Read the model definition and answer for the solid it produces. Units are mm, in the model's axes. Give positions to 0.01 mm unless a question says otherwise; leave off trailing zeros. Loops run counter-clockwise (first coordinate to the right, second up) from the corner with the lowest first, then second, coordinate; pieces in that order, holes last. Notation, with made-up numbers: (82.5, 41.5) - (108.5, 41.5) arc R15 ccw to (108.5, 67.5) - close; hole circle Ø3 at (16.5, 10). An arc over 180 degrees is marked (long way). Put each result on its own line as item: value. Start each with the question number.
1. A cutting plane is placed at C-C, the plane z = 51. Determine the outline of the cut face in (x, y).
2. Consider L1, parallel to Y at x = 0, z = 20; L2, parallel to Y at x = -8, z = 52; L3, parallel to X at y = -11, z = 26. Determine where each line is inside the solid, lowest interval first. Write a range as from..to.
3. Given pin 1 Ø5 at (y, z) = (-16.5, 18) entering from -X; pin 2 Ø10 at (y, z) = (15.5, 41) entering from +X; pin 3 Ø10 at (y, z) = (16, 10.5) entering from -X; pin 4 Ø4 at (x, y) = (16, -17.5) entering from +Z, each flat-ended and moving along its own axis, determine where each tip first touches the part or whether it passes through.
4. For a pull along X with two mould halves and no side action, classify faces 1 (the cylindrical face through (-4.336, -19.524, 32.115)), 2 (the cylindrical face through (-2.994, 22.804, 30.594)), 3 (the flat face through (-23.1, -2.2, 2)) as released by +X, released by -X, zero draft, split by the parting line, or undercut.
```python
from build123d import *

# Parameters (mm, degrees)
F0_R     = 23
F0_R_2   = 20
F1_DEPTH = 60
F0_R_3   = 31
F2_DEPTH = 2
F3_R     = 1.99999
F4_R     = 5


# Not quite as in the source:
# - a fillet or chamfer is up to 0.001 mm smaller than in the source, because OpenCascade refuses the exact size


with BuildPart() as f1:
    # F0 (on Top) → F1 (new body)
    with BuildSketch(Plane.XY):
        Circle(F0_R)
        Circle(F0_R_2, mode=Mode.SUBTRACT)
    extrude(amount=F1_DEPTH)

    # F0 (on Top) → F2 (join)
    with BuildSketch(Plane.XY):
        Circle(F0_R_3)
        Circle(F0_R, mode=Mode.SUBTRACT)
    extrude(amount=F2_DEPTH)

    # F3 (radius 2 in the source; OpenCascade refuses exactly that, so slightly less here)
    f3_edges = [f1.edges().sort_by_distance(p)[0] for p in [
        (-31, 0, 0),
    ]]
    fillet(f3_edges, radius=F3_R)

    # F4
    f4_edges = [f1.edges().sort_by_distance(p)[0] for p in [
        (-20, 0, 0),
    ]]
    fillet(f4_edges, radius=F4_R)


solid = f1.part
```
Return value:
1. outline: circle Ø46 at (0, 0); hole circle Ø40 at (0, 0)
2. L1: y = -23..-20, 20..23
2. L2: y = -21.56..-18.33, 18.33..21.56
2. L3: x = -20.2..-16.7, 16.7..20.2
3. pin 1: stops at x = -18.25
3. pin 2: stops at x = 20.46
3. pin 3: stops at x = -20.2
3. pin 4: stops at z = 60
4. face 1: undercut
4. face 2: split by the parting line
4. face 3: zero draft
